The model under review builds one solid part; all positions refer to its coordinate system, in mm. Face numbers are marked on the shaded views. A direction names the side the tool comes from. Round coordinates to 2 decimals unless told otherwise and drop trailing zeros. Order: outer loops, then holes, each group sorted by start corner. A loop starts at its lowest first (then second) coordinate and runs counter-clockwise, first axis right, second up.
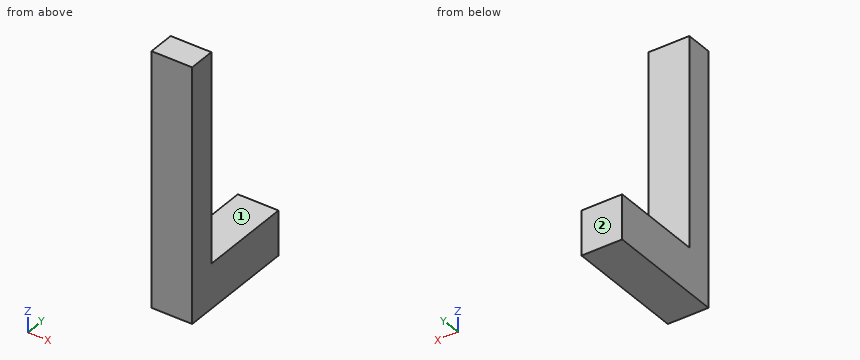
Autodesk Inventor part; units mm, degrees
ref_plane "YZ Plane" through (0, 0, 0) normal (1, 0, 0) x (0, 1, 0)
ref_plane "XZ Plane" through (0, 0, 0) normal (0, 1, 0) x (-1, 0, 0)
ref_plane "XY Plane" through (0, 0, 0) normal (0, 0, 1) x (1, 0, 0)
sketch "Sketch1" plane through (0, 0, 0) normal (0, 0, 1) x (1, 0, 0)
  line L0 (-2.6152, 0) -> (3.8148, 0)
  line L1 (3.8148, 0) -> (3.8148, 4.2707)
  line L2 (3.8148, 4.2707) -> (-2.6152, 4.2707)
  line L3 (-2.6152, 4.2707) -> (-2.6152, 0)
  point P0 (0, 0)
extrude "Extrusion1" add sketch "Sketch1" along normal blind 40
sketch "Sketch2" plane through (-2.6152, 4.2707, 0) normal (0, 1, 0) x (1, 0, 0)
  line L0 (0, 0) -> (0, -40)
  line L1 (0, -7.0299) -> (6.43, -7.0299)
  line L2 (6.43, -7.0299) -> (6.43, 0)
  line L3 (6.43, 0) -> (0, 0)
  line L4 (0, 0) -> (0, -7.0299)
  point P0 (2.6152, 0)
extrude "Extrusion2" add sketch "Sketch2" along normal blind 15
equation "\"BendRadius\" = Thickness"
equation "\"BendReliefWidth\" = Thickness"
equation "\"BendReliefDepth\" = 0.5 * Thickness"
equation "\"CornerReliefSize\" = 4 * Thickness"
equation "\"MinimumRemnant\" = 2 * Thickness"
equation "\"TransitionRadius\" = BendRadius"
equation "\"JacobiRadiusSize\" = BendRadius"
equation "\"GapSize\" = Thickness"
(1) Consider section A-A (x = -0.25). Write out the cut boundary in (y, z).
Data:
outline: (0, 0) - (19.27, 0) - (19.27, 7.03) - (4.27, 7.03) - (4.27, 40) - (0, 40) - close
(2) Insertion check: pin 1 (2 mm diameter, centred on x = -1, z = 11, fed in from +Y); pin 2 (1.9 mm diameter, centred on x = 0.5, y = 11.5, fed in from +Z). Each pin has a flat end and moves straight along its axis. Give the tip position at first contact, or say it passes through.
Data:
pin 1: stops at y = 4.27
pin 2: stops at z = 7.03
(3) For the marked faces 1 and 2, list the 3-axis set-ups (+Z, -Z, +X, -X, +Y, -Y) from which the entire face can be reached by the end or side of a thin tool; tool diameter is ignored.
Data:
face 1: +Z, +X, -X, +Y
face 2: +Z, -Z, +X, -X, +Y
(4) Consider section C-C (y = 12). Write out the cut boundary in (x, z), and give its area (3 significant figures).
Data:
outline: (-2.62, 0) - (3.81, 0) - (3.81, 7.03) - (-2.62, 7.03) - close
area: 45.2 mm2
(5) Consider section B-B (z = 10). Write out the cut boundary in (x, y).
Data:
outline: (-2.62, 0) - (3.81, 0) - (3.81, 4.27) - (-2.62, 4.27) - close
(6) To check wall thickness, follow probe 1 along Y at (x, z) = (-0.25, 35.5); probe 2 along Z at (x, y) = (-1.5, 13.25). State the ranges of each line that lie inside material, in increasing order.
Data:
probe 1: y = 0 to 4.27
probe 2: z = 0 to 7.03
